from build123d import *

# Parameters (mm, degrees)
F1_DEPTH  = 25.4
F3_DEPTH  = 82
F1_FACE_W = 25.4
F1_FACE_H = 31.75
F4_DEPTH  = 25.4
F5_W      = 12.7
F5_H      = 18.9845859185
F6_DEPTH  = 38.101
F8_DEPTH  = 25.4
F9_W      = 25.4
F9_H      = 12.7
F10_DEPTH = 0.254


# Not quite as in the source:
# - an extrude ends at something that could not be found from the text; its depth is read off the source's solid


with BuildPart() as f1:
    # F0 (on Front) → F1 (new body)
    with BuildSketch(Plane.XZ):
        Polygon((25.3994814964, 31.5877048481), (0, 31.75), (0, 0), (38.1, 0), (38.1, 12.7), align=None)
    extrude(amount=F1_DEPTH)

    # F2 (on Right) → F3 (cut, through all)
    with BuildSketch(Plane.YZ):
        Polygon((-12.9239121452, 31.9192558527), (-25.5880542099, 31.9192558527), (-25.4064481705, 12.6858642325), (-12.9239121452, 12.6858642325), align=None)
    extrude(amount=-F3_DEPTH, mode=Mode.SUBTRACT)

    # F2 (on Right) + F1_face (on face) → F4 (cut)
    with BuildSketch(Plane.YZ):
        Polygon((-12.9239121452, 31.9192558527), (-25.5880542099, 31.9192558527), (-25.4064481705, 12.6858642325), (-12.9239121452, 12.6858642325), align=None)
    with BuildSketch(Plane(origin=(0, -12.7, 15.875), x_dir=(0, -1, 0), z_dir=(-1, 0, 0))):
        Rectangle(F1_FACE_W, F1_FACE_H)
    extrude(amount=-F4_DEPTH, dir=(1, 0, 0), mode=Mode.SUBTRACT)

    # F5 (on face) → F6 (cut, through all)
    with BuildSketch(Plane(origin=(0, 0, 0), x_dir=(0, -1, 0), z_dir=(-1, 0, 0))):
        with Locations((19.05, 22.2577070408)):
            Rectangle(F5_W, F5_H)
    extrude(amount=-F6_DEPTH, mode=Mode.SUBTRACT)

    # F7 (on face) → F8 (cut)
    with BuildSketch(Plane.XY.offset(12.7654140815)):
        Polygon((38.056014097, -25.4), (38.056014097, -12.7), (30.7297278196, -25.4), align=None)
    extrude(amount=-F8_DEPTH, mode=Mode.SUBTRACT)

    # F9 (on face) → F10 (cut)
    with BuildSketch(Plane.YZ.offset(38.1)):
        with Locations((-12.7, 6.35)):
            Rectangle(F9_W, F9_H)
    extrude(amount=-F10_DEPTH, mode=Mode.SUBTRACT)


solid = f1.part
Build history of the part. All positions in model axes, mm. A direction names the side the tool comes from. Round coordinates to 2 decimals unless told otherwise and drop trailing zeros. Loops run counter-clockwise (first coordinate to the right, second up) from the corner with the lowest first, then second, coordinate; pieces in that order, holes last. Notation, with made-up numbers: (9, -7.5) -> (60, -7.5) arc R6 ccw to (60, 1.5) -> close; hole circle Ø3 at (29.5, -27.75). An arc over 180 degrees is marked (long way). One line per item, written item: value. Start each with the question number.
Q1. Drop flat-ended pins along their axis: pin 1 Ø6.5 at (y, z) = (-5, 6.5) entering from +X; pin 2 Ø1.5 at (x, y) = (25, -3.5) entering from +Z; pin 3 Ø4 at (x, y) = (15.5, -16.5) entering from +Z. Give the stop position or say it passes through.
Q2. Cut at A-A on y = -21. List the corners of the cut face in (x, z).
Q3. Cut at B-B on y = -4.75. List the corners of the cut face in (x, z).
Q4. Cut at C-C on x = 28.5. List the corners of the cut face in (y, z), plus the area to 3 significant figures.
Q5. Cut at D-D on y = -18. List the corners of the cut face in (x, z).
Q6. 3-axis set-ups, long thin cutter, end or side, ignore diameter. For faces 1 (the face through (15, -25.4, 6)), 2 (the face through (15, -12.7, 22)), 3 (the face through (37.846, -7, 6)): which of +Z, -Z, +X, -X, +Y, -Y reach the whole face in a straight line?
Q7. Probe line 1 along X through (y, z) = (-9.5, 3.5); line 2 along Z through (x, y) = (27.5, -20.5); line 3 along Y through (x, z) = (2.5, 30.5). List the from-to ranges inside material, lowest first.
Computed:
1. pin 1: x = 37.85
1. pin 2: z = 31.6
1. pin 3: z = 12.77
2. outline: (0, 0) -> (33.27, 0) -> (33.27, 12.77) -> (0, 12.77) -> close; (38.06, 12.7) -> (38.1, 12.7) -> (38.06, 12.77) -> close
3. outline: (0, 0) -> (37.85, 0) -> (37.85, 12.7) -> (38.1, 12.7) -> (25.4, 31.59) -> (0, 31.75) -> close
4. outline: (-25.4, 0) -> (0, 0) -> (0, 26.98) -> (-12.7, 26.98) -> (-12.7, 12.77) -> (-25.4, 12.77) -> close
4. area: 505 mm²
5. outline: (0, 0) -> (35, 0) -> (35, 12.77) -> (0, 12.77) -> close; (38.06, 12.7) -> (38.1, 12.7) -> (38.06, 12.77) -> close
6. face 1: +Z, -Z, +X, -X, -Y
6. face 2: +Z, +X, -X, -Y
6. face 3: -Z, +X, +Y, -Y
7. line 1: 0 to 37.85
7. line 2: 0 to 12.77
7. line 3: -12.7 to 0
